Here's the drawing with two shaded views (mm, measured from the low corner). I have some questions. A direction names the side the tool comes from. Round coordinates to 2 decimals unless told otherwise and drop trailing zeros. Write each loop counter-clockwise with the first axis right and the second up, starting at its lowest first coordinate (ties: lowest second). Pieces come first, ordered by that corner, then holes. Notation, with made-up numbers: M -30.75,14 L -16.75,14 A18 cw -16.75,46 Z; hole C 84,54 d5. An arc over 180 degrees is marked long. Write item = value, one per line. Start each with the question number.
(1) I want a section at D-D (z = 24.5). List the corners of the cut face in (x, y) for me, and give its area (3 significant figures).
(2) I need wall thicknesses on line 1 along Y through (x, z) = (5, 24.75); line 2 along Y through (x, z) = (19, 1.1). Which ranges of each line are inside material? Lowest first, please.
(3) I want a section at A-A (y = 33). List the corners of the cut face in (x, z) for me.
(4) I want a section at B-B (x = 19). List the corners of the cut face in (y, z) for me, and give its area (3 significant figures).
(5) On a 3-axis mill with a long thin cutter (end or side, diameter ignored), from which of +Z, -Z, +X, -X, +Y, -Y can I reach the whole of each face in a straight line? I mean the marked faces 5, 6 and 7. Say none if no direction works.
(6) If we mould it in two halves opening along X, with no side actions, what happens to the marked faces 1, 2, 3 and 4? For each: released by +X, released by -X, zero draft, split by the parting line, or undercut.
(7) Will these pins go through, and if not, where does the flat tip stop? pin 1 Ø8 at (x, y) = (33, 33) entering from -Z; pin 2 Ø12 at (y, z) = (31, 5.5) entering from +X; pin 3 Ø6 at (y, z) = (9.5, 6) entering from +X.
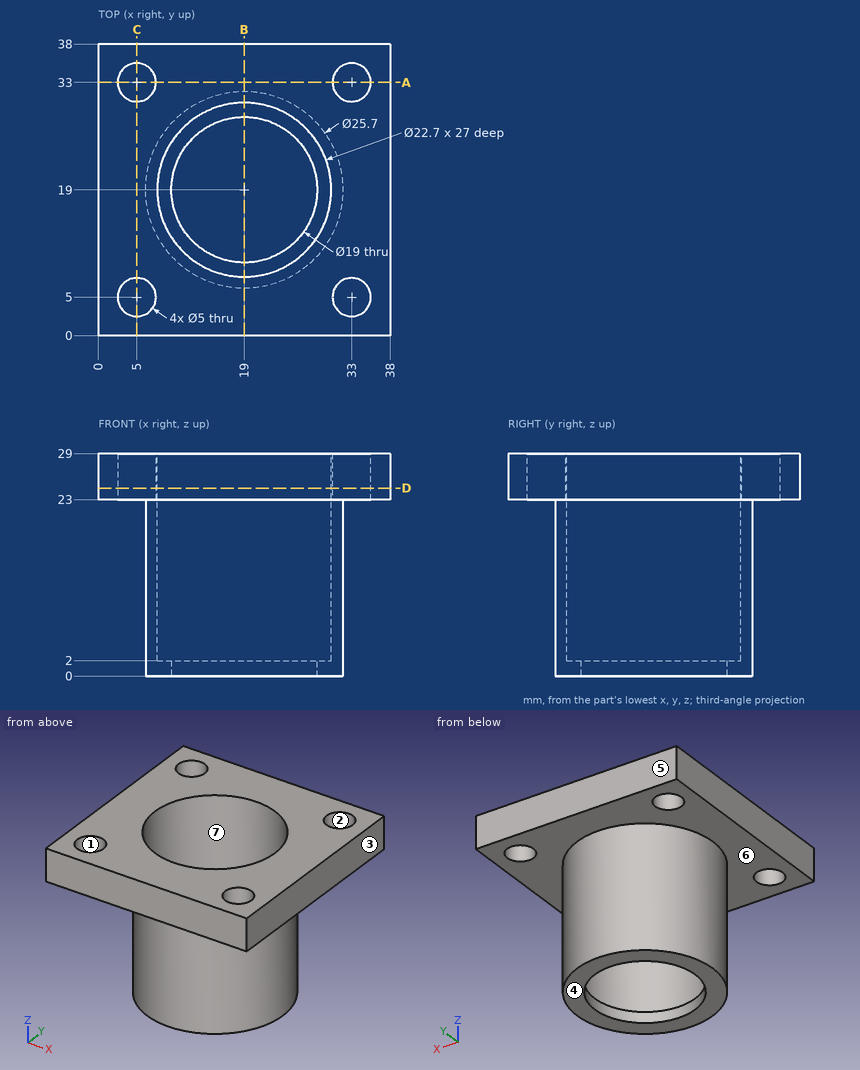
Returned:
q1.outline = M 0,0 L 38,0 L 38,38 L 0,38 Z; hole C 5,5 d5; hole C 5,33 d5; hole C 19,19 d22.7; hole C 33,5 d5; hole C 33,33 d5
q1.area = 961 mm²
q2.line_1 = 0 to 2.5, 7.5 to 30.5, 35.5 to 38
q2.line_2 = 6.15 to 9.5, 28.5 to 31.85
q3.outline = M 0,23 L 2.5,23 L 2.5,29 L 0,29 Z; M 7.5,23 L 30.5,23 L 30.5,29 L 7.5,29 Z; M 35.5,23 L 38,23 L 38,29 L 35.5,29 Z
q4.outline = M 0,23 L 6.15,23 L 6.15,0 L 9.5,0 L 9.5,2 L 7.65,2 L 7.65,29 L 0,29 Z; M 28.5,0 L 31.85,0 L 31.85,23 L 38,23 L 38,29 L 30.35,29 L 30.35,2 L 28.5,2 Z
q4.area = 168 mm²
q5.face_5 = +Z, -Z, +X, -X, +Y
q5.face_6 = -Z
q5.face_7 = +Z
q6.face_1 = undercut
q6.face_2 = undercut
q6.face_3 = released by +X
q6.face_4 = zero draft
q7.pin_1 = 23
q7.pin_2 = 30.36
q7.pin_3 = 30.08
